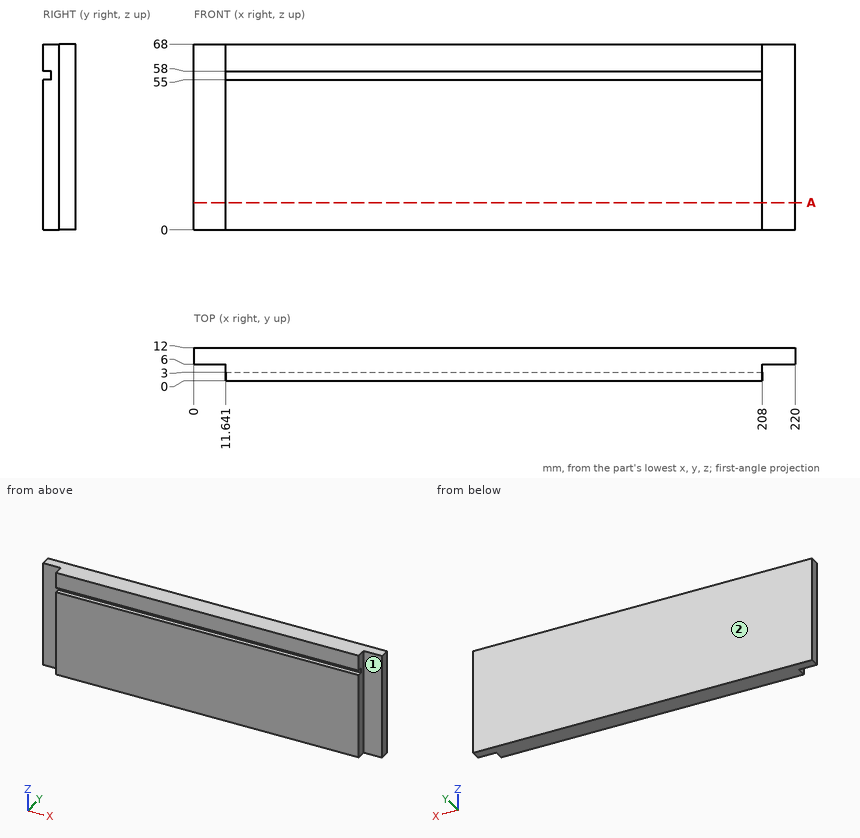
Print and shaded views of the part. All mm, measured from the part's lowest x, y and z. A direction names the side the tool comes from. Give positions to 0.01 mm unless a question says otherwise; leave off trailing zeros. Loops run counter-clockwise (first coordinate to the right, second up) from the corner with the lowest first, then second, coordinate; pieces in that order, holes last. Notation, with made-up numbers: (79, -22.75) -> (119, -22.75) arc R27 cw to (119, 11.25) -> close; hole circle Ø10 at (-28, 5.5). An arc over 180 degrees is marked (long way). Answer in a Markdown table with one row per item.
Item 1: Tool access for the marked faces 1 and 2: list every direction of +Z, -Z, +X, -X, +Y, -Y with a clear straight run to the whole face (end or side of a thin tool).
Findings below:
| item | result |
|---|---|
| face 1 | +Z, -Z, +X, -Y |
| face 2 | +Z, -Z, +X, -X, +Y |
Item 2: Probe line 1 along Z through (x, y) = (27.5, 2.75); line 2 along X through (y, z) = (0.5, 53.5). List the from-to ranges inside material, lowest first. Write a range as [from, to].
Findings below:
| item | result |
|---|---|
| line 1 | z = [0, 55], [58, 68] |
| line 2 | x = [11.64, 208] |
Item 3: Slice it at A-A on z = 10. Write the cut outline in (x, y), plus the area to 3 significant figures.
Findings below:
| item | result |
|---|---|
| outline | (0, 6) -> (11.64, 6) -> (11.64, 0) -> (208, 0) -> (208, 6) -> (220, 6) -> (220, 12) -> (0, 12) -> close |
| area | 2,500 mm² |
Item 4: Flat gauge pins, fed straight in: P1, Ø5, axis at y = 2.5, z = 37, coming from the +X side; P2, Ø6, axis at x = 211.5, z = 48, coming from the -Y side; P3, Ø3, axis at y = 3, z = 31, coming from the -X side. Where does each tip first touch, or does it go through?
Findings below:
| item | result |
|---|---|
| P1 | stops at x = 208 |
| P2 | stops at y = 6 |
| P3 | stops at x = 11.64 |
